```python
from build123d import *

# Parameters (mm, degrees)
F0_W     = 96.52
F0_H     = 5.08
F1_DEPTH = 40.64
F2_T     = -2.54
F3_W     = 48.26
F3_H     = 7.2280052118
F4_DEPTH = 5.081


with BuildPart() as f1:
    # F0 (on Front) → F1 (new body, symmetric)
    with BuildSketch(Plane.XZ):
        Rectangle(F0_W, F0_H)
    extrude(amount=F1_DEPTH, both=True)

    # F2
    f2_openings = [f1.faces().sort_by_distance(p)[0] for p in [
        (0, 0, 2.54),
    ]]
    offset(amount=F2_T, openings=f2_openings)

    # F3 (on face) → F4 (cut, through all)
    with BuildSketch(Plane(origin=(0, 0, -2.54), x_dir=(1, 0, 0), z_dir=(0, 0, -1))):
        with BuildLine():
            ThreePointArc((0, -3.6140026059), (3.6140026059, 0), (0, 3.6140026059))
            Line((0, 3.6140026059), (0, -3.6140026059))
        make_face()
        with Locations((-24.13, 0)):
            Rectangle(F3_W, F3_H)
    extrude(amount=-F4_DEPTH, mode=Mode.SUBTRACT)


solid = f1.part
```
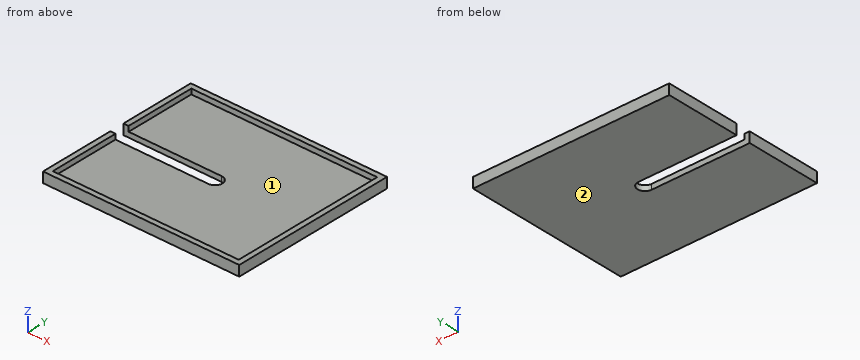
Geometry check sheet. Reference: the model listing, model coordinates, mm. Face numbers are marked on the shaded views. Coordinates: 2 decimals unless noted, no trailing zeros. Order: outer loops, then holes, each group sorted by start corner. A loop starts at its lowest first (then second) coordinate and runs counter-clockwise, first axis right, second up.
Item 1: Depth check by flat-ended pin: pin 1 (10 mm diameter, centred on x = 22, y = -9, fed in from +Z). Enter the tip coordinate at first touch or a pass-through.
Item 2: Section check D-D (y = 29). Enter the section's corners in (x, z), plus the area to 3 significant figures.
Item 3: Section check C-C (z = 1.5). Enter the section's corners in (x, y).
Item 4: Scan lines: line 1 along Y through (x, z) = (-10.5, -0.95); line 2 along Y through (x, z) = (43.5, 1.7); line 3 along X through (y, z) = (6.5, 0.25). Record each from-to range of solid material in increasing order.
Item 5: Mould release check, pull along Y, two halves, no side actions. Record for the marked faces 1 and 2: released by +Y, released by -Y, zero draft, split by the parting line, or undercut.
Item 6: Section check B-B (y = 0). Enter the section's corners in (x, z), plus the area to 3 significant figures.
Item 7: Section check A-A (x = -1.5). Enter the section's corners in (y, z), plus the area to 3 significant figures.
Check sheet entries:
1. pin 1: stops at z = 0
2. outline: (-48.26, -2.54) - (48.26, -2.54) - (48.26, 2.54) - (45.72, 2.54) - (45.72, 0) - (-45.72, 0) - (-45.72, 2.54) - (-48.26, 2.54) - close
2. area: 258 mm2
3. outline: (-48.26, -40.64) - (48.26, -40.64) - (48.26, 40.64) - (-48.26, 40.64) - (-48.26, 3.61) - (-45.72, 3.61) - (-45.72, 38.1) - (45.72, 38.1) - (45.72, -38.1) - (-45.72, -38.1) - (-45.72, -3.61) - (-48.26, -3.61) - close
4. line 1: y = -40.64 to -3.61, 3.61 to 40.64
4. line 2: y = -40.64 to -38.1, 38.1 to 40.64
4. line 3: x = -48.26 to -45.72, 45.72 to 48.26
5. face 1: undercut
5. face 2: zero draft
6. outline: (3.61, -2.54) - (48.26, -2.54) - (48.26, 2.54) - (45.72, 2.54) - (45.72, 0) - (3.61, 0) - close
6. area: 120 mm2
7. outline: (-40.64, -2.54) - (-3.61, -2.54) - (-3.61, 0) - (-38.1, 0) - (-38.1, 2.54) - (-40.64, 2.54) - close; (3.61, -2.54) - (40.64, -2.54) - (40.64, 2.54) - (38.1, 2.54) - (38.1, 0) - (3.61, 0) - close
7. area: 201 mm2
